Work out the finished part from the listing and answer in its coordinate system (mm). Face numbers are marked on the shaded views. A direction names the side the tool comes from. Round coordinates to 2 decimals unless told otherwise and drop trailing zeros. Write each loop counter-clockwise with the first axis right and the second up, starting at its lowest first coordinate (ties: lowest second). Pieces come first, ordered by that corner, then holes.
1. Find section D-D (z = -9.5). Write down the section's boundary in (x, y).
2. Find section B-B (x = -22.5). Write down the section's boundary in (y, z).
3. Find section C-C (z = 7.25). Write down the section's boundary in (x, y).
4. Find section A-A (y = -4). Write down the section's boundary in (x, z).
5. Determine the mould class of the marked faces 1, 2, 3 and 4 for opening direction X: pulls with the +X half, pulls with the -X half, needs draft (parallel to the pull), parting line crosses it, or undercut.
6. Straight lines are drawn through the part: probe 1 along Z at (x, y) = (52.5, -13); probe 2 along Z at (x, y) = (52, -13); probe 3 along X at (y, z) = (-28, -8.5). For each, find the intervals that lie inside material, in ascending order.
7. A tool of negligible diameter and unlimited length cuts with its end or side. For the marked faces 5, 6, 7, 8 and 9, from which of +Z, -Z, +X, -X, +Y, -Y can it reach the whole face along a straight path? Write none if from no direction.
8. Flat-ended cylindrical pins translate along their axes: pin 1 Ø10 at (x, z) = (34.5, -8) entering from +Y; pin 2 Ø1.5 at (x, z) = (-22, 0) entering from -Y; pin 3 Ø1.6 at (y, z) = (-34, -7.5) entering from +X; pin 4 Ø8 at (x, y) = (-50, -31) entering from +Z. Find the tip coordinate at first contact, or state that the pin passes through.
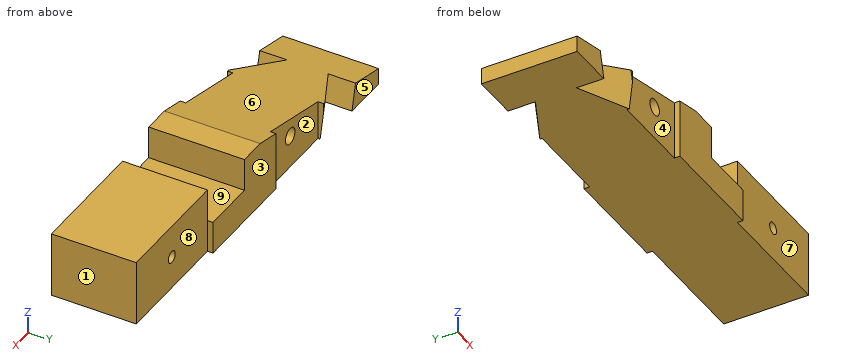
```python
from build123d import *

# Parameters (mm, degrees)
F0_W      = 150
F0_H      = 24
F0_R      = 3
F0_R_2    = 2.1592760918
F1_DEPTH  = 35
F3_DEPTH  = 35
F5_DEPTH  = 25
F6_W      = 20
F6_H      = 12
F7_DEPTH  = 35
F8_W      = 30
F8_H      = 2
F9_DEPTH  = 25
F10_W     = 45.1
F10_H     = 2
F11_DEPTH = 25


with BuildPart() as f1:
    # F0 (on Front) → F1 (new body)
    with BuildSketch(Plane.XZ):
        Rectangle(F0_W, F0_H)
        with Locations((-22.5, 0.0003034234)):
            Circle(F0_R, mode=Mode.SUBTRACT)
        with Locations((52.5, 0)):
            Circle(F0_R_2, mode=Mode.SUBTRACT)
    extrude(amount=F1_DEPTH)

    # F2 (on face) → F3 (cut)
    with BuildSketch(Plane.XZ.offset(35)):
        Polygon((-75, 12), (-75, -6), (0, 12), align=None)
    extrude(amount=-F3_DEPTH, mode=Mode.SUBTRACT)

    # F4 (on face) → F5 (cut)
    with BuildSketch(Plane(origin=(-2.7231467474, 0, 11.3464447806), x_dir=(0.972387302, 0, 0.2333729525), z_dir=(-0.2333729525, 0, 0.972387302))):
        Polygon((-59.3292853634, -25), (-59.3292853634, -35), (-39.3292853634, -35), align=None)
        Polygon((-39.3292853634, 0), (-59.3292853634, 0), (-59.3292853634, -10), align=None)
    extrude(amount=-F5_DEPTH, mode=Mode.SUBTRACT)

    # F6 (on face) → F7 (cut)
    with BuildSketch(Plane.XZ.offset(35)):
        with Locations((19.9226795137, 6)):
            Rectangle(F6_W, F6_H)
    extrude(amount=-F7_DEPTH, mode=Mode.SUBTRACT)

    # F8 (on face) → F9 (cut)
    with BuildSketch(Plane(origin=(0, 0, -12), x_dir=(1, 0, 0), z_dir=(0, 0, -1))):
        with Locations((-25, 34)):
            Rectangle(F8_W, F8_H)
        with Locations((-25, 1)):
            Rectangle(F8_W, F8_H)
    extrude(amount=-F9_DEPTH, mode=Mode.SUBTRACT)

    # F10 (on face) → F11 (cut)
    with BuildSketch(Plane(origin=(0, 0, -12), x_dir=(1, 0, 0), z_dir=(0, 0, -1))):
        with Locations((52.45, 34)):
            Rectangle(F10_W, F10_H)
        with Locations((52.45, 1)):
            Rectangle(F10_W, F10_H)
    extrude(amount=-F11_DEPTH, mode=Mode.SUBTRACT)


solid = f1.part
```
Worked answers:
1. outline: (-75, -35) - (-58.73, -35) - (-58.73, -25) - (-40, -34.11) - (-40, -33) - (-10, -33) - (-10, -35) - (29.9, -35) - (29.9, -33) - (75, -33) - (75, -2) - (29.9, -2) - (29.9, 0) - (-10, 0) - (-10, -2) - (-40, -2) - (-40, -0.89) - (-58.73, -10) - (-58.73, 0) - (-75, 0) - close
2. outline: (-33, -12) - (-2, -12) - (-2, -3) - (-33, -3) - close; (-33, 3) - (-2, 3) - (-2, 6.6) - (-33, 6.6) - close
3. outline: (-19.79, -33) - (-10, -33) - (-10, -35) - (9.92, -35) - (9.92, 0) - (-10, 0) - (-10, -2) - (-19.79, -2) - close; (29.92, -33) - (75, -33) - (75, -2) - (29.92, -2) - close
4. outline: (-75, -12) - (-58.13, -12) - (-60.41, -2.5) - (-75, -6) - close; (-48.75, 0.3) - (-45.79, -12) - (75, -12) - (75, 12) - (29.92, 12) - (29.92, 0) - (9.92, 0) - (9.92, 12) - (0, 12) - close; hole circle Ø6 at (-22.5, 0); hole circle Ø4.32 at (52.5, 0)
5. face 1: pulls with the +X half
5. face 2: undercut
5. face 3: needs draft
5. face 4: undercut
6. probe 1: z = -12 to -2.16, 2.16 to 12
6. probe 2: z = -12 to -2.1, 2.1 to 12
6. probe 3: x = -75 to -58.97, -52.8 to 75
7. face 5: +Z, -Z, +X, -X, +Y
7. face 6: +Z, -X, +Y, -Y
7. face 7: +Z, -Z, +X, -Y
7. face 8: +Z, -Z, +X, +Y
7. face 9: +Z, +Y, -Y
8. pin 1: stops at y = 0
8. pin 2: passes through
8. pin 3: stops at x = 29.9
8. pin 4: stops at z = 0.96
